For this review, take the finished solid that the model builds, in its own axes (mm). Face numbers are marked on the shaded views. A direction names the side the tool comes from. Coordinates: 2 decimals unless noted, no trailing zeros. Loops run counter-clockwise (first coordinate to the right, second up) from the corner with the lowest first, then second, coordinate; pieces in that order, holes last.
1. Take a section at A-A, the plane z = 5. State the section outline as (x, y) points, then the cut area to 3 significant figures.
2. Take a section at D-D, the plane y = 8. Count the separate pieces of the cut face and the enclosed holes in it, then the cut area to 3 significant figures.
3. Machinability: for the marked faces 5 and 6, which of the approach directions +Z, -Z, +X, -X, +Y, -Y give a long, thin tool a straight path to every point of the face, cutting with its end or side? Answer none if there is none.
4. To check wall thickness, follow probe 1 along Y at (x, z) = (22.65, 22.5); probe 2 along Y at (x, z) = (-22.35, 37.5); probe 3 along X at (y, z) = (0.5, 29.5). State the ranges of each line that lie inside material, in increasing order.
5. Take a section at C-C, the plane z = 27. State the section outline as (x, y) points, then the cut area to 3 significant figures.
6. Take a section at B-B, the plane y = -10. State the section outline as (x, z) points.
7. Clearance check with flat-ended pins moving along their axes: P1, Ø4.5, axis at y = -18, z = 22.5, coming from the -X side; P2, Ø3, axis at x = 7, z = 52.5, coming from the -Y side; P3, Ø12, axis at x = 12, z = 36.5, coming from the -Y side; P4, Ø2.5, axis at y = -18, z = 5, coming from the -X side. State where each tip first meets the part, or that it passes through.
8. Mouldability with a two-part tool opening along X and no side actions: class the marked faces 1, 2, 3 and 4 as pulls with the +X half, pulls with the -X half, needs draft (parallel to the pull), parting line crosses it, or undercut.
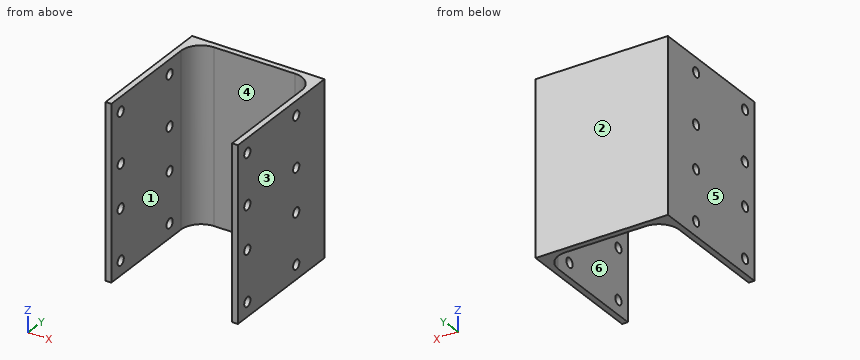
```python
from build123d import *

# Parameters (mm, degrees)
SKETCH_1_W                  = 46
SKETCH_1_H                  = 60
EXTRUDE_1_DEPTH             = 46
SKETCH_2_W                  = 42
SKETCH_2_H                  = 44
CUT_EXTRUDE_1_DEPTH         = 69.249542123
HOLE_WIZARD_3_3_3_3_1_D     = 3.3
HOLE_WIZARD_3_3_3_3_1_DEPTH = 2
HOLE_WIZARD_3_3_3_3_2_D     = 3.3
HOLE_WIZARD_3_3_3_3_2_DEPTH = 46
FILLET_1_R                  = 7


with BuildPart() as part:
    # 草图1 → 凸台-拉伸1 (new body)
    with BuildSketch(Plane.XZ.offset(23)):
        with Locations((0, 30)):
            Rectangle(SKETCH_1_W, SKETCH_1_H)
    extrude(amount=-EXTRUDE_1_DEPTH)

    # 草图2 → 切除-拉伸1 (cut, through all)
    with BuildSketch(Plane.XY.offset(60)):
        with Locations((0, -1)):
            Rectangle(SKETCH_2_W, SKETCH_2_H)
    extrude(amount=-CUT_EXTRUDE_1_DEPTH, mode=Mode.SUBTRACT)

    # Ø3.3 (3.3) 直径孔1
    with Locations(Plane.ZY.offset(23)):
        with Locations((55, -18), (22.5, -18), (22.5, 8), (55, 8), (5, 8), (37.5, 8), (37.5, -17.819824414), (5, -18)):
            Hole(HOLE_WIZARD_3_3_3_3_1_D / 2, depth=HOLE_WIZARD_3_3_3_3_1_DEPTH)

    # Ø3.3 (3.3) 直径孔2
    with Locations(Plane(origin=(23, 0, 0), x_dir=(0, 0, -1), z_dir=(1, 0, 0))):
        with Locations((-55, 8), (-22.5, 8), (-22.5, -18), (-55, -18), (-5, -18), (-5, 8), (-37.5, 8), (-37.5, -18)):
            Hole(HOLE_WIZARD_3_3_3_3_2_D / 2, depth=HOLE_WIZARD_3_3_3_3_2_DEPTH)

    # 圆角1
    fillet_1_edges = [part.edges().sort_by_distance(p)[0] for p in [
        (-21, 21, 30),
        (21, 21, 30),
    ]]
    fillet(fillet_1_edges, radius=FILLET_1_R)


solid = part.part
```
Results list:
1. outline: (-23, -23) - (-21, -23) - (-21, -19.65) - (-23, -19.65) - close; (-23, -16.35) - (-21, -16.35) - (-21, 6.35) - (-23, 6.35) - close; (-23, 9.65) - (-21, 9.65) - (-21, 14) arc R7 cw to (-14, 21) - (14, 21) arc R7 cw to (21, 14) - (21, 9.65) - (23, 9.65) - (23, 23) - (-23, 23) - close; (21, -23) - (23, -23) - (23, -19.65) - (21, -19.65) - close; (21, -16.35) - (23, -16.35) - (23, 6.35) - (21, 6.35) - close
1. area: 263 mm2
2. separate pieces: 10
2. enclosed holes: 0
2. area: 187 mm2
3. face 5: +Z, -Z, -X, +Y, -Y
3. face 6: +Z, -Z, -Y
4. probe 1: y = -23 to -19.65, -16.35 to 6.35, 9.65 to 23
4. probe 2: y = -23 to -19.65, -16.17 to 6.35, 9.65 to 23
4. probe 3: x = -23 to -21, 21 to 23
5. outline: (-23, -23) - (-21, -23) - (-21, 14) arc R7 cw to (-14, 21) - (14, 21) arc R7 cw to (21, 14) - (21, -23) - (23, -23) - (23, 23) - (-23, 23) - close
5. area: 289 mm2
6. outline: (-23, 0) - (-21, 0) - (-21, 60) - (-23, 60) - close; (21, 0) - (23, 0) - (23, 60) - (21, 60) - close
7. P1: stops at x = -23
7. P2: stops at y = 21
7. P3: stops at y = 19.74
7. P4: passes through
8. face 1: undercut
8. face 2: needs draft
8. face 3: pulls with the +X half
8. face 4: undercut
